```python
from build123d import *

# Parameters (mm, degrees)
SKETCH1_R               = 1.5
BOSS_EXTRUDE1_DEPTH     = 6
CUT_EXTRUDE1_DEPTH      = 7.97859592
CUT_EXTRUDE1_DEPTH_BACK = 7.97859592
CHAMFER1_SIZE           = 0.5


with BuildPart() as part:
    # Sketch1 → Boss-Extrude1 (new body)
    with BuildSketch(Plane(origin=(0, 0, 0), x_dir=(1, 0, 0), z_dir=(0, 1, 0))):
        with Locations(Location((0, 0, 0), (0, 0, 270))):
            Circle(SKETCH1_R)
    extrude(amount=BOSS_EXTRUDE1_DEPTH)

    # Sketch2 → Revolve1 (revolve)
    with BuildSketch(Plane.XY, mode=Mode.PRIVATE) as revolve1_sk:
        with BuildLine():
            Line((0, 0), (-2.52, 0))
            ThreePointArc((-2.52, 0), (-1.585449748, -1.440539697), (0, -2.1))
            Line((0, -2.1), (0, 0))
        make_face()
    revolve(revolve1_sk.sketch.rotate(Axis((0, -2.1, 0), (0, 1, 0)), 180), axis=Axis((0, -2.1, 0), (0, 1, 0)))

    # Sketch3 → Cut-Extrude1 (cut, two sides: drawn at the far end of the back side and taken through both)
    with BuildSketch(Plane.XY.offset(-CUT_EXTRUDE1_DEPTH_BACK)):
        Polygon((-0.5, -0.7), (0, -0.7), (0.5, -0.7), (0.5, -4.6380618), (-0.5, -4.6380618), align=None)
    extrude(amount=CUT_EXTRUDE1_DEPTH + CUT_EXTRUDE1_DEPTH_BACK, mode=Mode.SUBTRACT)

    # Chamfer1
    chamfer1_edges = [part.edges().sort_by_distance(p)[0] for p in [
        (0, 6, -1.5),
    ]]
    chamfer(chamfer1_edges, length=CHAMFER1_SIZE)


solid = part.part
```
Part model, mm, in its own coordinate system. A direction names the side the tool comes from. Round coordinates to 2 decimals unless told otherwise and drop trailing zeros.
Item 1: Drill centre lines: line 1 (X direction, y = -1, z = 0.4); line 2 (X direction, y = -1.25, z = -1.1); line 3 (Z direction, x = -0.05, y = 1.75). Where is each one in solid material? Low to high.
Item 2: 3-axis set-ups, long thin cutter, end or side, ignore diameter. For faces 1 (the face through (0.5, -1, 0)), 2 (the face through (0, 0, 2)): which of +Z, -Z, +X, -X, +Y, -Y reach the whole face in a straight line?
Item 3: Mould opens along X. For faces 3 (the face through (-0.5, -1, 0)), 4 (the face through (0, 6, 0)), 5 (the face through (0.45, 2.71, 1.43)), 6 (the face through (0, -0.7, 0)) say: +X half, -X half, draft (parallel to the pull), parting line (faces both ways), or undercut.
Item 4: Drop flat-ended pins along their axis: P1, Ø1, axis at y = -1, z = -2, coming from the -X side; P2, Ø2, axis at x = 1.5, y = 0, coming from the +Z side; P3, Ø0.7, axis at y = -1.5, z = 0.5, coming from the +X side. Give the stop position or say it passes through.
A:
1. line 1: x = -1.97 to -0.5, 0.5 to 1.97
1. line 2: x = -1.42 to -0.5, 0.5 to 1.42
1. line 3: z = -1.5 to 1.5
2. face 1: +Z, -Z, -Y
2. face 2: +Y
3. face 3: undercut
3. face 4: draft
3. face 5: parting line
3. face 6: undercut
4. P1: stops at x = -1.54
4. P2: stops at z = 2.47
4. P3: stops at x = 1.83
